The listing builds one solid part. Answer for the finished solid, in the listing's coordinates (mm). A direction names the side the tool comes from. Round coordinates to 2 decimals unless told otherwise and drop trailing zeros. Return JSON: item names as keys, results as strings. Group by question number.
(1) Each of these flat-tipped pins is pushed along its axis until it touches: pin 1 (2.5 mm diameter, centred on y = 58.5, z = -4, fed in from -X); pin 2 (3 mm diameter, centred on x = 12, z = -4, fed in from -Y). Where does it stop, or does it pass through?
(2) Consider line 1 (X direction, y = -71, z = -4); line 2 (Y direction, x = 7.25, z = -4); line 3 (Z direction, x = 12, y = -67). Determine where each line is inside the solid, lowest interval first. Write a range as [from, to].
(3) Which of the six approach directions +Z, -Z, +X, -X, +Y, -Y give full straight-line access (tool end or side, diameter ignored) to faces 4 (the face through (5.12, 0.07, -2.35)), 5 (the face through (13, 70.56, -5.31)), 6 (the face through (58, -70.56, -5.31))?
(4) Determine the mould class of faces 1 (the face through (13, -70.56, -5.31)), 2 (the face through (2.5, 76, -3.9)), 3 (the face through (34, 1, 0)) for opening direction X: +X half, -X half, draft (parallel to the pull), parting line (faces both ways), or undercut.
from build123d import *

# Parameters (mm, degrees)
SKETCH1_W                      = 68
SKETCH1_H                      = 157
BOSS_EXTRUDE1_DEPTH            = 8
M4X0_7_TAPPED_HOLE1_AT_2_COUNT = 2
M4X0_7_TAPPED_HOLE1_AT_2_PITCH = 45
M4X0_7_TAPPED_HOLE2_D          = 3.3
M4X0_7_TAPPED_HOLE2_DEPTH      = 10.1
M4X0_7_TAPPED_HOLE2_TIP        = 0.991420021
CHAMFER1_SIZE                  = 5


with BuildPart() as part:
    # Sketch1 → Boss-Extrude1 (new body)
    with BuildSketch(Plane.XY):
        with Locations((34, 0)):
            Rectangle(SKETCH1_W, SKETCH1_H)
    extrude(amount=-BOSS_EXTRUDE1_DEPTH)

    # Sketch4 → M4x0.7 Tapped Hole1 (revolve, cut)
    with BuildSketch(Plane(origin=(12, 78.5, -4), x_dir=(0, 0, 1), z_dir=(1, 0, 0))):
        Polygon((0, 0), (0, 17.091420021), (1.65, 16.1), (1.65, 0), align=None)
    m4x0_7_tapped_hole1 = revolve(axis=Axis((12, 84.85, -4), (0, -1, 0)), mode=Mode.SUBTRACT)

    # M4x0.7 Tapped Hole1 at 2: M4x0.7 Tapped Hole1 ×2
    with Locations(*[(i * M4X0_7_TAPPED_HOLE1_AT_2_PITCH, 0, 0) for i in range(1, M4X0_7_TAPPED_HOLE1_AT_2_COUNT)]):
        add(m4x0_7_tapped_hole1, mode=Mode.SUBTRACT)

    # M4x0.7 Tapped Hole2
    with Locations(Plane.ZY):
        with Locations((-4, 58.5), (-4, 0), (-4, -58.5)):
            Hole(M4X0_7_TAPPED_HOLE2_D / 2, depth=M4X0_7_TAPPED_HOLE2_DEPTH)
            with Locations((0, 0, -(M4X0_7_TAPPED_HOLE2_DEPTH + M4X0_7_TAPPED_HOLE2_TIP / 2))):  # 118° drill point
                Cone(0, M4X0_7_TAPPED_HOLE2_D / 2, M4X0_7_TAPPED_HOLE2_TIP, mode=Mode.SUBTRACT)

    # Mirror1: M4x0.7 Tapped Hole1 across plane
    add(m4x0_7_tapped_hole1.mirror(Plane.ZX), mode=Mode.SUBTRACT)

    # Mirror1 copy 1 sketch → Mirror1 copy 1 (revolve, cut)
    with BuildSketch(Plane(origin=(57, -78.5, -4), x_dir=(0, 0, 1), z_dir=(1, 0, 0))):
        Polygon((0, 0), (0, -17.091420021), (1.65, -16.1), (1.65, 0), align=None)
    revolve(axis=Axis((57, -84.85, -4), (0, -1, 0)), mode=Mode.SUBTRACT)

    # Chamfer1
    chamfer1_edges = [part.edges().sort_by_distance(p)[0] for p in [
        (0, -78.5, -4),
        (0, 78.5, -4),
    ]]
    chamfer(chamfer1_edges, length=CHAMFER1_SIZE)


solid = part.part
Answer below:
{
 "1": {"pin 1": "stops at x = 10.34", "pin 2": "stops at y = -62.31"},
 "2": {"line 1": "x = [0, 10.35], [13.65, 55.35], [58.65, 68]", "line 2": "y = [-78.5, -60.15], [-56.85, -1.65], [1.65, 56.85], [60.15, 78.5]", "line 3": "z = [-8, -5.65], [-2.35, 0]"},
 "3": {"face 4": "-X", "face 5": "+Y", "face 6": "-Y"},
 "4": {"face 1": "undercut", "face 2": "-X half", "face 3": "draft"}
}
